Geometry check sheet. Reference: the model listing, model coordinates, mm. Face numbers are marked on the shaded views. A direction names the side the tool comes from. Give positions to 0.01 mm unless a question says otherwise; leave off trailing zeros. Loops run counter-clockwise (first coordinate to the right, second up) from the corner with the lowest first, then second, coordinate; pieces in that order, holes last. Notation, with made-up numbers: (-3.5, -18) -> (1.5, -18) arc R12 ccw to (1.5, 0) -> close; hole circle Ø3 at (-3.5, -32). An arc over 180 degrees is marked (long way). One line per item, written item: value. Start each with the question number.
(1) Sectioned sample at A-A, the plane y = 1. Record the cut outline in (x, z), then the cut area to 3 significant figures.
(2) Sectioned sample at C-C, the plane z = 2.5. Record the cut outline in (x, y).
(3) Sectioned sample at D-D, the plane y = 2. Record the cut outline in (x, z), then the cut area to 3 significant figures.
(4) Scan lines: line 1 along Y through (x, z) = (2.3, -3); line 2 along Z through (x, y) = (0, 0.95); line 3 along Y through (x, z) = (-1.4, -3). Record each from-to range of solid material in increasing order. Write a range as from..to.
(5) Tool access check on the marked faces 5, 6, 7 and 8. Record the directions out of +Z, -Z, +X, -X, +Y, -Y that give a thin tool (end or side, any length) a straight path to the whole face; none if there is none.
(6) Gauge pin test, flat ends, axial feed: pin 1 Ø2 at (x, z) = (0, -2.5) entering from -Y; pin 2 Ø1.5 at (x, z) = (-0.5, -3.5) entering from +Y; pin 3 Ø2 at (x, y) = (-1, 4) entering from -Z. Record the tip position at first contact, or that the pin passes through.
(7) Sectioned sample at B-B, the plane x = 0. Record the cut outline in (y, z).
(8) Draft check along Z on the marked faces 1, 2, 3 and 4. Enter one of: pulls with the +Z half, pulls with the -Z half, needs draft (parallel to the pull), parting line crosses it, or undercut.
Autodesk Inventor part; units mm, degrees
ref_plane "YZ Plane" through (0, 0, 0) normal (1, 0, 0) x (0, 1, 0)
ref_plane "XZ Plane" through (0, 0, 0) normal (0, 1, 0) x (-1, 0, 0)
ref_plane "XY Plane" through (0, 0, 0) normal (0, 0, 1) x (1, 0, 0)
sketch "草圖1" plane through (0, 0, 0) normal (0, 1, 0) x (-1, 0, 0)
  line L0 (2.5, 5) -> (-2.5, 5)
  line L1 (-2.5, 5) -> (-2.5, -5)
  line L2 (-2.5, -5) -> (2.5, -5)
  line L3 (2.5, -5) -> (2.5, 5)
  circle A0 centre (0, 2.5) radius 1.7
  circle A1 centre (0, -2.5) radius 1.7
  line L4 (2.5, 0) -> (-2.5, 0)
  point P0 (0, 0)
  point P1 (0, -5)
  dimension "d0" = 5
  dimension "d1" = 10
  dimension "d2" = 3.4
  dimension "d3" = 3.4
  dimension "d4" = 2.5
  dimension "d5" = 2.5
  dimension "d6" = 2.5
  dimension "d7" = 2.5
extrude "擠出1" add sketch "草圖1" along normal blind 2.5 contours L3 L2 L1 L4 | A1
extrude "擠出2" cut sketch "草圖1" along normal blind 1.5 contours A1
sketch "草圖2" plane through (0, 2.5, 0) normal (0, 1, 0) x (1, 0, 0)
  circle A0 centre (0, 2.5) radius 1.7
  point P0 (0, 0)
extrude "擠出3" add sketch "草圖2" along normal blind 1.5
sketch "草圖3" plane through (0, 0, 0) normal (1, 0, 0) x (0, 1, 0)
  line L0 (0, 5) -> (0, -5)
  line L1 (0, 0) -> (5, 5)
  line L2 (5, 5) -> (5, 0)
  line L3 (5, 0) -> (0, 0)
  dimension "d15" = 5
  dimension "d20" = 5
extrude "擠出4" add sketch "草圖3" along normal mid plane 5
sketch "草圖4" plane through (-2.5, 5, 5) normal (0, 1, 0) x (1, 0, 0)
  circle A0 centre (2.5, 2.5) radius 1.7
  point P0 (2.5, 5)
extrude "擠出5" add sketch "草圖4" along normal blind 1.5
properties part number "110033226_ipt_11_樓梯支架"
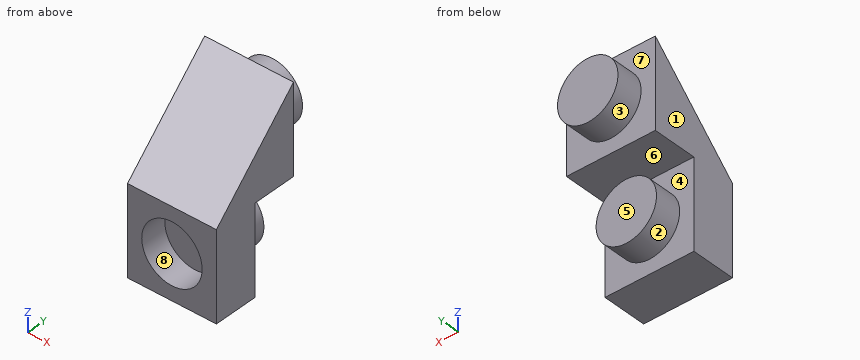
Calculated:
1. outline: (-2.5, -5) -> (2.5, -5) -> (2.5, 1) -> (-2.5, 1) -> close; hole circle Ø3.4 at (0, -2.5)
1. area: 20.9 mm2
2. outline: (-2.5, 2.5) -> (2.5, 2.5) -> (2.5, 5) -> (1.7, 5) -> (1.7, 6.5) -> (-1.7, 6.5) -> (-1.7, 5) -> (-2.5, 5) -> close
3. outline: (-2.5, -5) -> (2.5, -5) -> (2.5, 2) -> (-2.5, 2) -> close
3. area: 35.0 mm2
4. line 1: y = 0..2.5
4. line 2: z = -5..-4.2, -0.8..0.95
4. line 3: y = 1.5..4
5. face 5: -Z, +X, -X, +Y
5. face 6: +X, -X, +Y
5. face 7: +Y
5. face 8: -Y
6. pin 1: stops at y = 1.5
6. pin 2: stops at y = 4
6. pin 3: stops at z = -4.2
7. outline: (0, -5) -> (2.5, -5) -> (2.5, -4.2) -> (4, -4.2) -> (4, -0.8) -> (2.5, -0.8) -> (2.5, 0) -> (5, 0) -> (5, 0.8) -> (6.5, 0.8) -> (6.5, 4.2) -> (5, 4.2) -> (5, 5) -> (0, 0) -> (0, -0.8) -> (1.5, -0.8) -> (1.5, -4.2) -> (0, -4.2) -> close
8. face 1: needs draft
8. face 2: undercut
8. face 3: parting line crosses it
8. face 4: undercut
